Design review of the part built by this model. Coordinates are the model's own, in mm. Face numbers are marked on the shaded views. A direction names the side the tool comes from. Give positions to 0.01 mm unless a question says otherwise; leave off trailing zeros. Write each loop counter-clockwise with the first axis right and the second up, starting at its lowest first coordinate (ties: lowest second). Pieces come first, ordered by that corner, then holes. Notation, with made-up numbers: M -38,51 L 18,51 A22 cw 18,81 Z; hole C 68.25,-6 d4. An arc over 180 degrees is marked long. Answer in a Markdown table with one row per item.
```python
from build123d import *

# Parameters (mm, degrees)
F0_R     = 6.5
F0_R_2   = 2.25
F1_DEPTH = 35
F3_D     = 2.2
F7_DEPTH = 10


with BuildPart() as f1:
    # F0 (on Top) → F1 (new body)
    with BuildSketch(Plane.XY):
        Circle(F0_R)
        Circle(F0_R_2, mode=Mode.SUBTRACT)
    extrude(amount=F1_DEPTH)

    # F3 (through all)
    with Locations(Plane(origin=(0, 0, 0), x_dir=(1, 0, 0), z_dir=(0, 0, -1))):
        with Locations((0, -4.75), (0, 4.75)):
            Hole(F3_D / 2)

    # F6 (on offset) → F7 (cut)
    with BuildSketch(Plane(origin=(0, 0, 3), x_dir=(1, 0, 0), z_dir=(0, 0, -1))):
        with BuildLine():
            Line((2, -6.75), (2, -4.75))
            ThreePointArc((2, -4.75), (0, -2.75), (-2, -4.75))
            Line((-2, -4.75), (-2, -6.75))
            Line((-2, -6.75), (2, -6.75))
        make_face()
    extrude(amount=-F7_DEPTH, mode=Mode.SUBTRACT)


solid = f1.part
```
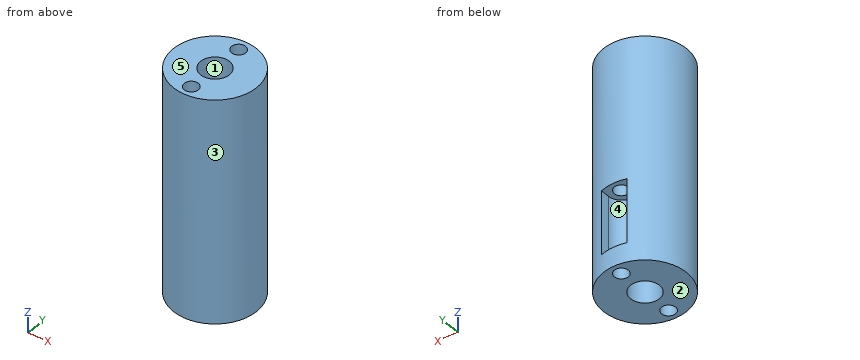
1) The part is to be moulded in two halves that separate along X. For the marked faces 1, 2 and 3, say which applies: released by +X, released by -X, zero draft, split by the parting line, or undercut.
Geometry says:
| item | result |
|---|---|
| face 1 | undercut |
| face 2 | zero draft |
| face 3 | split by the parting line |
2) Add section C-C (z = 21). Write out the cut boundary in (x, y).
Geometry says:
| item | result |
|---|---|
| outline | C 0,0 d13; hole C 0,0 d4.5; hole C 0,-4.75 d2.2; hole C 0,4.75 d2.2 |
3) Add section A-A (x = 0). Write out the cut boundary in (y, z).
Geometry says:
| item | result |
|---|---|
| outline | M -6.5,0 L -5.85,0 L -5.85,35 L -6.5,35 Z; M -3.65,0 L -2.25,0 L -2.25,35 L -3.65,35 Z; M 2.25,0 L 3.65,0 L 3.65,3 L 2.75,3 L 2.75,13 L 3.65,13 L 3.65,35 L 2.25,35 Z; M 5.85,0 L 6.5,0 L 6.5,3 L 5.85,3 Z; M 5.85,13 L 6.5,13 L 6.5,35 L 5.85,35 Z |
4) Add section B-B (y = 0). Write out the cut boundary in (x, z).
Geometry says:
| item | result |
|---|---|
| outline | M -6.5,0 L -2.25,0 L -2.25,35 L -6.5,35 Z; M 2.25,0 L 6.5,0 L 6.5,35 L 2.25,35 Z |
5) Insertion check: P1, Ø1.1, axis at y = 5, z = 9, coming from the -X side; P2, Ø2, axis at x = 0, y = 4.75, coming from the -Z side; P3, Ø3, axis at y = 3, z = 24, coming from the -X side; P4, Ø1, axis at x = -5, z = 15.5, coming from the -Y side. Each pin has a flat end and moves straight along its axis. Give the tip position at first contact, or say it passes through.
Geometry says:
| item | result |
|---|---|
| P1 | x = -4.74 |
| P2 | through |
| P3 | x = -6.32 |
| P4 | y = -4.69 |
6) For the marked faces 4 and 5, list the 3-axis set-ups (+Z, -Z, +X, -X, +Y, -Y) from which the entire face can be reached by the end or side of a thin tool; tool diameter is ignored.
Geometry says:
| item | result |
|---|---|
| face 4 | +Y |
| face 5 | +Z, +X, -X, +Y, -Y |
7) Add section D-D (y = 3.25). Write out the cut boundary in (x, z).
Geometry says:
| item | result |
|---|---|
| outline | M -5.63,0 L 5.63,0 L 5.63,35 L -5.63,35 Z; hole M -1.32,3 L 1.32,3 L 1.32,13 L -1.32,13 Z |
8) To check wall thickness, follow probe 1 along Y at (x, z) = (0, 29); probe 2 along Y at (x, z) = (0, 10.5); probe 3 along X at (y, z) = (-4.25, 21). State the ranges of each line that lie inside material, in increasing order. Write a range as [from, to].
Geometry says:
| item | result |
|---|---|
| probe 1 | [-6.5, -5.85], [-3.65, -2.25], [2.25, 3.65], [5.85, 6.5] |
| probe 2 | [-6.5, -5.85], [-3.65, -2.25], [2.25, 2.75] |
| probe 3 | [-4.92, -0.98], [0.98, 4.92] |
